Read the model definition and answer for the solid it produces. Units are mm, in the model's axes. A direction names the side the tool comes from. Coordinates: 2 decimals unless noted, no trailing zeros. Order: outer loops, then holes, each group sorted by start corner. A loop starts at its lowest first (then second) coordinate and runs counter-clockwise, first axis right, second up.
```python
from build123d import *

# Parameters (mm, degrees)
BOSS_EXTRUDE1_DEPTH = 5.08
CUT_EXTRUDE1_DEPTH  = 1.27
SKETCH4_R           = 1.905
CUT_EXTRUDE2_DEPTH  = 7.62
SKETCH5_R           = 1.905
SKETCH5_W           = 88.9
SKETCH5_H           = 19.05
CUT_EXTRUDE3_DEPTH  = 7.62
SKETCH7_R           = 6.35
CUT_EXTRUDE5_DEPTH  = 7.62
SKETCH8_R           = 1.5
CUT_EXTRUDE6_DEPTH  = 25.4
SKETCH9_R           = 2
CUT_EXTRUDE7_DEPTH  = 381
SKETCH10_R          = 1.4224
CUT_EXTRUDE8_DEPTH  = 12.7
SKETCH6_R           = 6.35
CUT_EXTRUDE9_DEPTH  = 5.08
SKETCH11_R          = 1.1303
CUT_EXTRUDE10_DEPTH = 438.831463922


with BuildPart() as part:
    # Sketch2 → Boss-Extrude1 (new body)
    with BuildSketch(Plane.XY):
        Polygon((0, 0), (32.101676515, 0), (141.594783791, 130.488803961), (263.277562057, 0), (373.38, 0), (373.38, 228.6), (0, 228.6), align=None)
    extrude(amount=BOSS_EXTRUDE1_DEPTH)

    # Sketch3 → Cut-Extrude1 (cut)
    with BuildSketch(Plane.XY.offset(5.08)):
        Polygon((13.716, 0), (24.372565316, 0), (141.594783791, 139.7), (271.867141325, 0), (283.710082919, 0), (141.594783791, 152.4), align=None)
    extrude(amount=-CUT_EXTRUDE1_DEPTH, mode=Mode.SUBTRACT)

    # Sketch4 → Cut-Extrude2 (cut)
    with BuildSketch(Plane.XY.offset(3.81)):
        with Locations((51.69789323, 38.91505771)):
            Circle(SKETCH4_R)
        with Locations((84.351503802, 77.830115421)):
            Circle(SKETCH4_R)
        with Locations((117.005114374, 116.745173131)):
            Circle(SKETCH4_R)
        with Locations((167.57892131, 118.185423968)):
            Circle(SKETCH4_R)
        with Locations((242.932920113, 37.378153476)):
            Circle(SKETCH4_R)
        with Locations((260.255678459, 18.801769455)):
            Circle(SKETCH4_R)
    extrude(amount=-CUT_EXTRUDE2_DEPTH, mode=Mode.SUBTRACT)

    # Sketch5 → Cut-Extrude3 (cut)
    with BuildSketch(Plane.XY.offset(5.08)):
        with Locations((30.48, 212.598)):
            Circle(SKETCH5_R)
        with Locations((132.08, 212.598)):
            Circle(SKETCH5_R)
        with Locations((30.48, 161.798)):
            Circle(SKETCH5_R)
        with Locations((132.08, 161.798)):
            Circle(SKETCH5_R)
        with Locations((81.28, 203.073)):
            Rectangle(SKETCH5_W, SKETCH5_H)
    extrude(amount=-CUT_EXTRUDE3_DEPTH, mode=Mode.SUBTRACT)

    # Sketch7 → Cut-Extrude5 (cut)
    with BuildSketch(Plane.XY.offset(5.08)):
        with Locations((309.88, 107.95)):
            Circle(SKETCH7_R)
        with Locations((63.5, 107.95)):
            Circle(SKETCH7_R)
    extrude(amount=-CUT_EXTRUDE5_DEPTH, mode=Mode.SUBTRACT)

    # Sketch8 → Cut-Extrude6 (cut)
    with BuildSketch(Plane.XY.offset(5.08)):
        with Locations((2.54, 218.44)):
            Circle(SKETCH8_R)
        with Locations((218.44, 218.44)):
            Circle(SKETCH8_R)
        with Locations((281.94, 218.44)):
            Circle(SKETCH8_R)
        with Locations((345.44, 218.44)):
            Circle(SKETCH8_R)
    extrude(amount=-CUT_EXTRUDE6_DEPTH, mode=Mode.SUBTRACT)

    # Sketch9 → Cut-Extrude7 (cut)
    with BuildSketch(Plane.XY.offset(5.08)):
        with Locations((322.58, 132.08)):
            Circle(SKETCH9_R)
        with Locations((271.78, 132.08)):
            Circle(SKETCH9_R)
        with Locations((220.98, 132.08)):
            Circle(SKETCH9_R)
        with Locations((119.38, 132.08)):
            Circle(SKETCH9_R)
        with Locations((68.58, 132.08)):
            Circle(SKETCH9_R)
    extrude(amount=-CUT_EXTRUDE7_DEPTH, mode=Mode.SUBTRACT)

    # Sketch10 → Cut-Extrude8 (cut)
    with BuildSketch(Plane(origin=(373.38, 0, 0), x_dir=(0, 0, -1), z_dir=(1, 0, 0))):
        with Locations((-2.54, 203.2)):
            Circle(SKETCH10_R)
        with Locations((-2.54, 156.21)):
            Circle(SKETCH10_R)
    extrude(amount=-CUT_EXTRUDE8_DEPTH, mode=Mode.SUBTRACT)

    # Sketch6 → Cut-Extrude9 (cut)
    with BuildSketch(Plane.XY.offset(5.08)):
        with Locations((212.494293851, 169.478312144)):
            Circle(SKETCH6_R)
        with Locations((280.053051399, 97.030414462)):
            Circle(SKETCH6_R)
        with Locations((327.886055199, 10.284305918)):
            Circle(SKETCH6_R)
    extrude(amount=-CUT_EXTRUDE9_DEPTH, mode=Mode.SUBTRACT)

    # Sketch11 → Cut-Extrude10 (cut, through all)
    with BuildSketch(Plane(origin=(0, 0, 0), x_dir=(-1, 0, 0), z_dir=(0, 0, -1))):
        with Locations((-316.75973092, 63.088723784)):
            Circle(SKETCH11_R)
        with Locations((-250.246994693, 62.340329973)):
            Circle(SKETCH11_R)
        with Locations((-283.511442727, 42.644318593)):
            Circle(SKETCH11_R)
    extrude(amount=-CUT_EXTRUDE10_DEPTH, mode=Mode.SUBTRACT)


solid = part.part
```
1) Determine the mould class of faces 4 (the flat face through (184, 141, 0)), 5 (the flat face through (205.819, 70.828, 4.454)), 6 (the flat face through (201.58, 66.16, 2.5)) for opening direction Y: pulls with the +Y half, pulls with the -Y half, needs draft (parallel to the pull), parting line crosses it, or undercut.
A:
face 4: needs draft
face 5: undercut
face 6: pulls with the -Y half
2) A cutting plane is placed at D-D, the plane z = 2.54. State how many separate pieces and enclosed holes the cut face has, and give its area (3 significant figures).
A:
separate pieces: 1
enclosed holes: 28
area: 67,700 mm2
3) A cutting plane is placed at C-C, the plane x = 189. Determine the outline of the cut face in (y, z), and give its area (3 significant figures).
A:
outline: (79.65, 0) - (228.6, 0) - (228.6, 5.08) - (101.56, 5.08) - (101.56, 3.81) - (88.86, 3.81) - (88.86, 5.08) - (79.65, 5.08) - close
area: 741 mm2
4) Straight lines are drawn through the part: line 1 (Y direction, x = 30.48, z = 2.95); line 2 (X direction, y = 208, z = 0.65); line 3 (X direction, y = 218, z = 3.1). For each, find the intervals that lie inside material, in ascending order.
A:
line 1: y = 0 to 159.89, 163.7 to 210.69, 214.5 to 228.6
line 2: x = 0 to 36.83, 125.73 to 373.38
line 3: x = 0 to 1.11, 3.97 to 217.01, 219.87 to 280.51, 283.37 to 344.01, 346.87 to 373.38
5) A flat-ended cylindrical pin translates along its axis: pin 1 Ø2 at (x, z) = (93, 0.5) entering from -Y. Find the tip coordinate at first contact, or state that the pin passes through.
A:
pin 1: stops at y = 71.38
6) A cutting plane is placed at A-A, the plane y = 125. Determine the outline of the cut face in (x, z).
A:
outline: (0, 0) - (136.99, 0) - (136.99, 5.08) - (129.26, 5.08) - (129.26, 3.81) - (118.6, 3.81) - (118.6, 5.08) - (0, 5.08) - close; (146.71, 0) - (373.38, 0) - (373.38, 5.08) - (167.15, 5.08) - (167.15, 3.81) - (155.3, 3.81) - (155.3, 5.08) - (146.71, 5.08) - close
7) Which of the six approach directions +Z, -Z, +X, -X, +Y, -Y give full straight-line access (tool end or side, diameter ignored) to faces 1 (the flat face through (213.65, 75.13, 4.45)), 2 (the flat face through (86.08, 64.33, 2.5)), 3 (the cylindrical face through (303.536, 108.229, 2.576))?
A:
face 1: +Z
face 2: +Z, -Z, -Y
face 3: +Z, -Z
8) A cutting plane is placed at B-B, the plane x = 309.88. Determine the outline of the cut face in (y, z), and give its area (3 significant figures).
A:
outline: (0, 0) - (101.6, 0) - (101.6, 5.08) - (0, 5.08) - close; (114.3, 0) - (228.6, 0) - (228.6, 5.08) - (114.3, 5.08) - close
area: 1,100 mm2
